from build123d import *

# Parameters (mm, degrees)
F0_W            = 52
F0_H            = 41
F1_DEPTH        = 10
F3_DEPTH        = 20
F4_R            = 11
F5_DEPTH        = 10.001
F6_R            = 15
F7_DEPTH        = 5
F9_R            = 3
F10_R           = 11.5
F10_R_2         = 9.5
F11_DEPTH       = 35
F12_T3_DEPTH    = 35
F12_T5_DEPTH    = 46
F12_T8_ANGLE    = 90
F12_T10_ANGLE   = 90
F12_T12_ANGLE   = 90
F12_T14_ANGLE   = 90
F13_R           = 10
F14_DEPTH       = 32
F15_R           = 11.5
F16_DEPTH       = 32
F18_D           = 3
F18_CSINK_D     = 6
F18_CSINK_ANGLE = 90


# Not quite as in the source:
# - a fillet or chamfer that OpenCascade refuses, or shapes differently, is made with other operations: its cross-section is extruded or revolved along the edge and cut away or added


with BuildPart() as f1:
    # F0 (on Top) → F1 (new body)
    with BuildSketch(Plane.XY):
        with Locations((26, 20.5)):
            Rectangle(F0_W, F0_H)
    extrude(amount=F1_DEPTH)

    # F2 (on face) → F3 (join)
    with BuildSketch(Plane.XY.offset(10)):
        with BuildLine():
            ThreePointArc((41, 19), (15.3933982822, 29.6066017178), (26, 4))
            ThreePointArc((26, 4), (36.6066017178, 8.3933982822), (41, 19))
        make_face()
        with BuildLine():
            ThreePointArc((37, 19), (33.7781745931, 11.2218254069), (26, 8))
            ThreePointArc((26, 8), (18.2218254069, 26.7781745931), (37, 19))
        make_face(mode=Mode.SUBTRACT)
    extrude(amount=F3_DEPTH)

    # F4 (on face) → F5 (cut, through all)
    with BuildSketch(Plane.XY.offset(10)):
        with Locations((26, 19)):
            Circle(F4_R)
    extrude(amount=-F5_DEPTH, mode=Mode.SUBTRACT)

    # F6 (on face) → F7 (join)
    with BuildSketch(Plane.XY.offset(30)):
        with Locations((26, 19)):
            Circle(F6_R)
    extrude(amount=F7_DEPTH)

    # F8: fillet of radius 2 on 1 edges, made by hand

    # F8_s1 → F8_t2 (revolve, cut)
    with BuildSketch(Plane.XZ.offset(-19)):
        with BuildLine():
            ThreePointArc((41, 33), (40.4142135624, 34.4142135624), (39, 35))
            Line((39, 35), (41, 35))
            Line((41, 35), (41, 33))
        make_face()
    revolve(axis=Axis((26, 19, 35), (0, 0, 1)), mode=Mode.SUBTRACT)

    # F9
    f9_edges = [f1.edges().sort_by_distance(p)[0] for p in [
        (52, 0, 5),
        (0, 0, 5),
        (0, 41, 5),
        (52, 41, 5),
    ]]
    fillet(f9_edges, radius=F9_R)

    # F10 (on face) → F11 (join)
    with BuildSketch(Plane(origin=(0, 0, 0), x_dir=(1, 0, 0), z_dir=(0, 0, -1))):
        with Locations((26, -19)):
            Circle(F10_R)
        with Locations((26, -19)):
            Circle(F10_R_2, mode=Mode.SUBTRACT)
    extrude(amount=-F11_DEPTH)

    # F12: fillet of radius 2 on 9 edges, made by hand

    # F12_s1 → F12_t2 (revolve)
    with BuildSketch(Plane.YZ.offset(26)):
        with BuildLine():
            ThreePointArc((1.9990343146, 9.9996), (3.4142135624, 10.5857864376), (4.0004, 12.0009656854))
            Line((4.0004, 12.0009656854), (4.2005365685, 12.0009656854))
            ThreePointArc((4.2005365685, 12.0009656854), (4.2001365685, 11.0004828427), (4.2001365685, 10))
            Line((4.2001365685, 10), (4, 9.7998634315))
            ThreePointArc((4, 9.7998634315), (2.9995171573, 9.7998634315), (1.9990343146, 9.7994634315))
            Line((1.9990343146, 9.7994634315), (1.9990343146, 9.9996))
        make_face()
    revolve(axis=Axis((26, 19, 10), (0, 0, 1)))

    # F12_s4 → F12_t3 (cut)
    with BuildSketch(Plane.XZ.offset(-38)):
        with BuildLine():
            ThreePointArc((-0.0004, 7.9990343146), (0.5857864376, 9.4142135624), (2.0009656854, 10.0004))
            Line((2.0009656854, 10.0004), (2.0009656854, 10.2005365685))
            ThreePointArc((2.0009656854, 10.2005365685), (1.0004828427, 10.2001365685), (0, 10.2001365685))
            Line((0, 10.2001365685), (-0.2001365685, 10))
            ThreePointArc((-0.2001365685, 10), (-0.2001365685, 8.9995171573), (-0.2005365685, 7.9990343146))
            Line((-0.2005365685, 7.9990343146), (-0.0004, 7.9990343146))
        make_face()
        with BuildLine():
            ThreePointArc((49.9990343146, 10.0004), (51.4142135624, 9.4142135624), (52.0004, 7.9990343146))
            Line((52.0004, 7.9990343146), (52.2005365685, 7.9990343146))
            ThreePointArc((52.2005365685, 7.9990343146), (52.2001365685, 8.9995171573), (52.2001365685, 10))
            Line((52.2001365685, 10), (52, 10.2001365685))
            ThreePointArc((52, 10.2001365685), (50.9995171573, 10.2001365685), (49.9990343146, 10.2005365685))
            Line((49.9990343146, 10.2005365685), (49.9990343146, 10.0004))
        make_face()
    extrude(amount=F12_T3_DEPTH, mode=Mode.SUBTRACT)

    # F12_s6 → F12_t5 (cut)
    with BuildSketch(Plane.YZ.offset(3)):
        with BuildLine():
            ThreePointArc((38.9990343146, 10.0004), (40.4142135624, 9.4142135624), (41.0004, 7.9990343146))
            Line((41.0004, 7.9990343146), (41.2005365685, 7.9990343146))
            ThreePointArc((41.2005365685, 7.9990343146), (41.2001365685, 8.9995171573), (41.2001365685, 10))
            Line((41.2001365685, 10), (41, 10.2001365685))
            ThreePointArc((41, 10.2001365685), (39.9995171573, 10.2001365685), (38.9990343146, 10.2005365685))
            Line((38.9990343146, 10.2005365685), (38.9990343146, 10.0004))
        make_face()
        with BuildLine():
            ThreePointArc((2.0009656854, 10.0004), (0.5857864376, 9.4142135624), (-0.0004, 7.9990343146))
            Line((-0.0004, 7.9990343146), (-0.2005365685, 7.9990343146))
            ThreePointArc((-0.2005365685, 7.9990343146), (-0.2001365685, 8.9995171573), (-0.2001365685, 10))
            Line((-0.2001365685, 10), (0, 10.2001365685))
            ThreePointArc((0, 10.2001365685), (1.0004828427, 10.2001365685), (2.0009656854, 10.2005365685))
            Line((2.0009656854, 10.2005365685), (2.0009656854, 10.0004))
        make_face()
    extrude(amount=F12_T5_DEPTH, mode=Mode.SUBTRACT)

    # F12_s7 → F12_t8 (revolve, cut)
    with BuildSketch(Plane.XZ.offset(-38)):
        with BuildLine():
            ThreePointArc((2.0009656854, 10.0004), (0.5857864376, 9.4142135624), (-0.0004, 7.9990343146))
            Line((-0.0004, 7.9990343146), (-0.2005365685, 7.9990343146))
            ThreePointArc((-0.2005365685, 7.9990343146), (-0.2001365685, 8.9995171573), (-0.2001365685, 10))
            Line((-0.2001365685, 10), (0, 10.2001365685))
            ThreePointArc((0, 10.2001365685), (1.0004828427, 10.2001365685), (2.0009656854, 10.2005365685))
            Line((2.0009656854, 10.2005365685), (2.0009656854, 10.0004))
        make_face()
    revolve(axis=Axis((3, 38, 10), (0, 0, -1)), revolution_arc=F12_T8_ANGLE, mode=Mode.SUBTRACT)

    # F12_s9 → F12_t10 (revolve, cut)
    with BuildSketch(Plane.XZ.offset(-3)):
        with BuildLine():
            ThreePointArc((2.0009656854, 10.0004), (0.5857864376, 9.4142135624), (-0.0004, 7.9990343146))
            Line((-0.0004, 7.9990343146), (-0.2005365685, 7.9990343146))
            ThreePointArc((-0.2005365685, 7.9990343146), (-0.2001365685, 8.9995171573), (-0.2001365685, 10))
            Line((-0.2001365685, 10), (0, 10.2001365685))
            ThreePointArc((0, 10.2001365685), (1.0004828427, 10.2001365685), (2.0009656854, 10.2005365685))
            Line((2.0009656854, 10.2005365685), (2.0009656854, 10.0004))
        make_face()
    revolve(axis=Axis((3, 3, 10), (0, 0, 1)), revolution_arc=F12_T10_ANGLE, mode=Mode.SUBTRACT)

    # F12_s11 → F12_t12 (revolve, cut)
    with BuildSketch(Plane.YZ.offset(49)):
        with BuildLine():
            ThreePointArc((38.9990343146, 10.0004), (40.4142135624, 9.4142135624), (41.0004, 7.9990343146))
            Line((41.0004, 7.9990343146), (41.2005365685, 7.9990343146))
            ThreePointArc((41.2005365685, 7.9990343146), (41.2001365685, 8.9995171573), (41.2001365685, 10))
            Line((41.2001365685, 10), (41, 10.2001365685))
            ThreePointArc((41, 10.2001365685), (39.9995171573, 10.2001365685), (38.9990343146, 10.2005365685))
            Line((38.9990343146, 10.2005365685), (38.9990343146, 10.0004))
        make_face()
    revolve(axis=Axis((49, 38, 10), (0, 0, -1)), revolution_arc=F12_T12_ANGLE, mode=Mode.SUBTRACT)

    # F12_s13 → F12_t14 (revolve, cut)
    with BuildSketch(Plane.YZ.offset(49)):
        with BuildLine():
            ThreePointArc((2.0009656854, 10.0004), (0.5857864376, 9.4142135624), (-0.0004, 7.9990343146))
            Line((-0.0004, 7.9990343146), (-0.2005365685, 7.9990343146))
            ThreePointArc((-0.2005365685, 7.9990343146), (-0.2001365685, 8.9995171573), (-0.2001365685, 10))
            Line((-0.2001365685, 10), (0, 10.2001365685))
            ThreePointArc((0, 10.2001365685), (1.0004828427, 10.2001365685), (2.0009656854, 10.2005365685))
            Line((2.0009656854, 10.2005365685), (2.0009656854, 10.0004))
        make_face()
    revolve(axis=Axis((49, 3, 10), (0, 0, 1)), revolution_arc=F12_T14_ANGLE, mode=Mode.SUBTRACT)

    # F13 (on face) → F14 (cut)
    with BuildSketch(Plane(origin=(0, 0, 0), x_dir=(1, 0, 0), z_dir=(0, 0, -1))):
        with Locations((26, -19)):
            Circle(F13_R)
    extrude(amount=-F14_DEPTH, mode=Mode.SUBTRACT)

    # F15 (on face) → F16 (cut, through all)
    with BuildSketch(Plane(origin=(0, 0, 0), x_dir=(1, 0, 0), z_dir=(0, 0, -1))):
        with Locations((26, -19)):
            Circle(F15_R)
    extrude(amount=-F16_DEPTH, mode=Mode.SUBTRACT)

    # F18 (through all)
    with Locations(Plane.XY.offset(35)):
        with Locations((26, 19)):
            CounterSinkHole(F18_D / 2, F18_CSINK_D / 2, counter_sink_angle=F18_CSINK_ANGLE)


solid = f1.part
Can you work these out from the model? Positions are in its coordinate system, mm. A direction names the side the tool comes from. Give positions to 0.01 mm unless a question says otherwise; leave off trailing zeros. Order: outer loops, then holes, each group sorted by start corner. A loop starts at its lowest first (then second) coordinate and runs counter-clockwise, first axis right, second up. Notation, with made-up numbers: M 5,-0.5 L 42,-0.5 A20 cw 42,5.5 Z; hole C -2,67 d2. An arc over 180 degrees is marked long. One line per item, written item: value.
Item 1: For faces 5 (the face through (0.57, 20.74, 9.4)), 6 (the face through (26, 37, 10)), which set-ups out of +Z, -Z, +X, -X, +Y, -Y let a thin tool reach every point of the face, with its end or its side?
Verdict:
face 5: +Z, -X, +Y, -Y
face 6: +Z
Item 2: If we section it at A-A on z = 5: Write out the boundary of the cut face in (x, y), and give its area (3 significant figures).
Verdict:
outline: M 0,3 A3 ccw 3,0 L 49,0 A3 ccw 52,3 L 52,38 A3 ccw 49,41 L 3,41 A3 ccw 0,38 Z; hole C 26,19 d23
area: 1,710 mm2
Item 3: For pin 1 (4 mm diameter, centred on x = 26, y = 19, fed in from -Z); pin 2 (3 mm diameter, centred on y = 30.5, z = 20, fed in from +X); pin 3 (6 mm diameter, centred on x = 11, y = 6.5, fed in from +Z), each with a flat end and sliding along its axis, tell me the tip position at first contact or that it passes through.
Verdict:
pin 1: z = 32
pin 2: x = 37.18
pin 3: z = 10.06
Item 4: Please list where these lines run through material, in increasing order: line 1 (Y direction, x = 26, z = 19); line 2 (X direction, y = 19, z = 29); line 3 (Y direction, x = 26, z = 33.2).
Verdict:
line 1: 4 to 7.5, 30.5 to 34
line 2: 11 to 14.5, 37.5 to 41
line 3: 4.01 to 17.5, 20.5 to 33.99
Item 5: If we mould it in two halves opening along X, with no side actions, what happens to faces 1 (the face through (51.4, 20.74, 9.43)), 2 (the face through (26, 17, 34)), 3 (the face through (0.86, 0.9, 4.08)), 4 (the face through (27.11, 20.01, 32.74))? For each: pulls with the +X half, pulls with the -X half, needs draft (parallel to the pull), parting line crosses it, or undercut.
Verdict:
face 1: pulls with the +X half
face 2: undercut
face 3: pulls with the -X half
face 4: undercut
Item 6: If we section it at B-B on x = 44.5: Write out the boundary of the cut face in (y, z), and give its area (3 significant figures).
Verdict:
outline: M 0,0 L 41,0 L 41,8.04 A2 ccw 39.04,10 L 1.96,10 A2 ccw 0,8.04 Z
area: 408 mm2
Item 7: If we section it at C-C on z = 21: Write out the boundary of the cut face in (x, y), and give its area (3 significant figures).
Verdict:
outline: C 26,19 d30; hole C 26,19 d23
area: 291 mm2
